from build123d import *

# Parameters (mm, degrees)
ESQUISSE1_W           = 161.925
ESQUISSE1_H           = 161.925
ESQUISSE1_R           = 39.6875
BOSS_EXTRU_1_DEPTH    = 19.05
TROU_TARAUD_3_8_161_D = 7.9375


with BuildPart() as part:
    # Esquisse1 → Boss.-Extru.1 (new body)
    with BuildSketch(Plane(origin=(0, 0, 0), x_dir=(1, 0, 0), z_dir=(0, 1, 0))):
        Rectangle(ESQUISSE1_W, ESQUISSE1_H)
        Circle(ESQUISSE1_R, mode=Mode.SUBTRACT)
        with BuildLine():
            ThreePointArc((-46.438182228, 66.320597386), (-57.249132772, 57.249132772), (-66.320597386, 46.438182228))
            ThreePointArc((-66.320597386, 46.438182228), (-64.371340998, 35.383399913), (-53.316558683, 37.332656301))
            ThreePointArc((-53.316558683, 37.332656301), (-46.02381262, 46.02381262), (-37.332656301, 53.316558683))
            ThreePointArc((-37.332656301, 53.316558683), (-35.383399913, 64.371340998), (-46.438182228, 66.320597386))
        make_face(mode=Mode.SUBTRACT)
        with BuildLine():
            ThreePointArc((66.320597386, 46.438182228), (57.249132772, 57.249132772), (46.438182228, 66.320597386))
            ThreePointArc((46.438182228, 66.320597386), (35.383399913, 64.371340998), (37.332656301, 53.316558683))
            ThreePointArc((37.332656301, 53.316558683), (46.02381262, 46.02381262), (53.316558683, 37.332656301))
            ThreePointArc((53.316558683, 37.332656301), (64.371340998, 35.383399913), (66.320597386, 46.438182228))
        make_face(mode=Mode.SUBTRACT)
        with BuildLine():
            ThreePointArc((46.438182228, -66.320597386), (57.249132772, -57.249132772), (66.320597386, -46.438182228))
            ThreePointArc((66.320597386, -46.438182228), (64.371340998, -35.383399913), (53.316558683, -37.332656301))
            ThreePointArc((53.316558683, -37.332656301), (46.02381262, -46.02381262), (37.332656301, -53.316558683))
            ThreePointArc((37.332656301, -53.316558683), (35.383399913, -64.371340998), (46.438182228, -66.320597386))
        make_face(mode=Mode.SUBTRACT)
        with BuildLine():
            ThreePointArc((-66.320597386, -46.438182228), (-57.249132772, -57.249132772), (-46.438182228, -66.320597386))
            ThreePointArc((-46.438182228, -66.320597386), (-35.383399913, -64.371340998), (-37.332656301, -53.316558683))
            ThreePointArc((-37.332656301, -53.316558683), (-46.02381262, -46.02381262), (-53.316558683, -37.332656301))
            ThreePointArc((-53.316558683, -37.332656301), (-64.371340998, -35.383399913), (-66.320597386, -46.438182228))
        make_face(mode=Mode.SUBTRACT)
    extrude(amount=-BOSS_EXTRU_1_DEPTH)

    # Trou taraudé 3/8-161 (through all)
    with Locations(Plane(origin=(0, 0, 0), x_dir=(1, 0, 0), z_dir=(0, 1, 0))):
        with Locations((-63.5, 63.5), (63.5, 63.5), (-63.5, -63.5), (63.5, -63.5)):
            Hole(TROU_TARAUD_3_8_161_D / 2)


solid = part.part
Part model, mm, in its own coordinate system. Give positions to 0.01 mm unless a question says otherwise; leave off trailing zeros. Order: outer loops, then holes, each group sorted by start corner. A loop starts at its lowest first (then second) coordinate and runs counter-clockwise, first axis right, second up. Notation, with made-up numbers: (-40, 77.5) - (-35, 77.5) arc R22 cw to (-35, 93.5) - close; hole circle Ø5 at (64, -35.75). An arc over 180 degrees is marked (long way). Use a Markdown table: item, result.
1) Saw through at B-B on x = 0. List the corners of the cut face in (y, z), plus the area to 3 significant figures.
Checked values:
| item | result |
|---|---|
| outline | (-19.05, -80.96) - (0, -80.96) - (0, -39.69) - (-19.05, -39.69) - close; (-19.05, 39.69) - (0, 39.69) - (0, 80.96) - (-19.05, 80.96) - close |
| area | 1,570 mm² |
2) Saw through at C-C on z = -22. List the corners of the cut face in (x, y).
Checked values:
| item | result |
|---|---|
| outline | (-80.96, -19.05) - (-33.03, -19.05) - (-33.03, 0) - (-80.96, 0) - close; (33.03, -19.05) - (80.96, -19.05) - (80.96, 0) - (33.03, 0) - close |
3) Flat gauge pin, fed straight in: P1, Ø5, axis at x = 63.5, z = -63.5, coming from the -Y side. Where does the tip first touch, or does it go through?
Checked values:
| item | result |
|---|---|
| P1 | through |
4) Two-plate mould, pull along Z, no slides. Class faces 1 (the cylindrical face through (35.485, -9.392, -64.513)), 2 (the flat face through (-1, -9, -80.962)), 3 (the flat face through (80.962, -9, 1)): +Z half, -Z half, draft (parallel to the pull), parting line (faces both ways), or undercut.
Checked values:
| item | result |
|---|---|
| face 1 | undercut |
| face 2 | -Z half |
| face 3 | draft |
5) Saw through at D-D on x = 64. List the corners of the cut face in (y, z).
Checked values:
| item | result |
|---|---|
| outline | (-19.05, -80.96) - (0, -80.96) - (0, -67.44) - (-19.05, -67.44) - close; (-19.05, -59.56) - (0, -59.56) - (0, -49.59) - (-19.05, -49.59) - close; (-19.05, -35.14) - (0, -35.14) - (0, 35.14) - (-19.05, 35.14) - close; (-19.05, 49.59) - (0, 49.59) - (0, 59.56) - (-19.05, 59.56) - close; (-19.05, 67.44) - (0, 67.44) - (0, 80.96) - (-19.05, 80.96) - close |
6) Probe L1, parallel to X at y = -6, z = 0; L2, parallel to X at y = -9.75, z = 63.5; L3, parallel to X at y = -7.75, z = -36. List the from-to ranges inside material, lowest first. Write a range as from..to.
Checked values:
| item | result |
|---|---|
| L1 | -80.96..-39.69, 39.69..80.96 |
| L2 | -80.96..-67.47, -59.53..-50.23, -34.85..34.85, 50.23..59.53, 67.47..80.96 |
| L3 | -80.96..-65.14, -54.49..-16.71, 16.71..54.49, 65.14..80.96 |
7) Saw through at A-A on y = -15.25. Count the separate pieces of the cut face and the enclosed holes in it, plus the area to 3 significant figures.
Checked values:
| item | result |
|---|---|
| separate pieces | 1 |
| enclosed holes | 9 |
| area | 18,700 mm² |
